from build123d import *

# Parameters (mm, degrees)
SKETCH1_W           = 80
SKETCH1_H           = 80
BOSS_EXTRUDE1_DEPTH = 5
SKETCH2_W           = 80
SKETCH2_H           = 5
BOSS_EXTRUDE2_DEPTH = 82
CUT_EXTRUDE1_DEPTH  = 81
CUT_EXTRUDE2_DEPTH  = 6
FILLET1_R           = 5
FILLET2_R           = 5
BOSS_EXTRUDE3_DEPTH = 80


with BuildPart() as part:
    # Sketch1 → Boss-Extrude1 (new body)
    with BuildSketch(Plane(origin=(0, 0, 0), x_dir=(1, 0, 0), z_dir=(0, 1, 0))):
        Rectangle(SKETCH1_W, SKETCH1_H)
    extrude(amount=BOSS_EXTRUDE1_DEPTH)

    # Sketch2 → Boss-Extrude2 (add)
    with BuildSketch(Plane(origin=(0, 5, 0), x_dir=(1, 0, 0), z_dir=(0, 1, 0))):
        with Locations((0, 37.5)):
            Rectangle(SKETCH2_W, SKETCH2_H)
    extrude(amount=BOSS_EXTRUDE2_DEPTH)

    # Sketch6 → Cut-Extrude1 (cut, through all)
    with BuildSketch(Plane(origin=(0, 0, -40), x_dir=(-1, 0, 0), z_dir=(0, 0, -1))):
        with BuildLine():
            Line((-30, 82), (30, 82))
            ThreePointArc((30, 82), (35, 77), (30, 72))
            Line((30, 72), (-30, 72))
            ThreePointArc((-30, 72), (-35, 77), (-30, 82))
        make_face()
        with BuildLine():
            Line((-30, 57), (30, 57))
            ThreePointArc((30, 57), (35, 52), (30, 47))
            Line((30, 47), (-30, 47))
            ThreePointArc((-30, 47), (-35, 52), (-30, 57))
        make_face()
    extrude(amount=-CUT_EXTRUDE1_DEPTH, mode=Mode.SUBTRACT)

    # Sketch7 → Cut-Extrude2 (cut, through all)
    with BuildSketch(Plane(origin=(0, 5, 0), x_dir=(1, 0, 0), z_dir=(0, 1, 0))):
        with BuildLine():
            Line((-35, -30), (-35, 15))
            ThreePointArc((-35, 15), (-30, 20), (-25, 15))
            Line((-25, 15), (-25, -30))
            ThreePointArc((-25, -30), (-30, -35), (-35, -30))
        make_face()
        with BuildLine():
            Line((35, 15), (35, -30))
            ThreePointArc((35, -30), (30, -35), (25, -30))
            Line((25, -30), (25, 15))
            ThreePointArc((25, 15), (30, 20), (35, 15))
        make_face()
    extrude(amount=-CUT_EXTRUDE2_DEPTH, mode=Mode.SUBTRACT)

    # Fillet1
    fillet1_edges = [part.edges().sort_by_distance(p)[0] for p in [
        (40, 2.5, 40),
        (-40, 2.5, 40),
    ]]
    fillet(fillet1_edges, radius=FILLET1_R)

    # Fillet2
    fillet2_edges = [part.edges().sort_by_distance(p)[0] for p in [
        (-40, 87, -37.5),
        (40, 87, -37.5),
    ]]
    fillet(fillet2_edges, radius=FILLET2_R)

    # Sketch8 → Boss-Extrude3 (add)
    with BuildSketch(Plane(origin=(40, 0, 0), x_dir=(0, 0, -1), z_dir=(1, 0, 0))):
        Polygon((35, 15), (25, 5), (35, 5), align=None)
    extrude(amount=-BOSS_EXTRUDE3_DEPTH)


solid = part.part
Check sheet for the modelled part. Datum: model origin and axes. Units: mm. A direction names the side the tool comes from. Round coordinates to 2 decimals unless told otherwise and drop trailing zeros. Write each loop counter-clockwise with the first axis right and the second up, starting at its lowest first coordinate (ties: lowest second). Pieces come first, ordered by that corner, then holes. Notation, with made-up numbers: (33, -12.75) -> (92, -12.75) arc R23 ccw to (92, 26.25) -> close; hole circle Ø1 at (76.25, 42). An arc over 180 degrees is marked (long way). Answer as CSV lines item,"result". Start each with the question number.
1) Section check D-D on x = 28.5. Enter the section's corners in (y, z).
2) Material ranges on line 1 (Z direction, x = -18, y = 61.5); line 2 (Y direction, x = 8, z = -0.5); line 3 (Y direction, x = -2, z = -28), recorded low to high. Write a range as from..to.
3) Tool access check on faces 5 (the flat face through (-35, 3, 8)), 6 (the flat face through (0, 82, -38)), 7 (the cylindrical face through (38, 86, -38)). Record the directions out of +Z, -Z, +X, -X, +Y, -Y that give a thin tool (end or side, any length) a straight path to the whole face; none if there is none.
4) Section check C-C on y = 52. Enter the section's corners in (x, z).
5) Section check B-B on z = 3.5. Enter the section's corners in (x, y).
6) Release check for a two-part mould opening along Z. For faces 1 (the cylindrical face through (30, 3, 35)), 2 (the flat face through (-1, 33, -40)), 3 (the flat face through (-25, 3, 7)), 4 (the flat face through (0, 47, -38)) record: pulls with the +Z half, pulls with the -Z half, needs draft (parallel to the pull), parting line crosses it, or undercut.
7) Section check A-A on x = -4.5. Enter the section's corners in (y, z), and give its area (3 significant figures).
8) Go/stop test with a flat-tipped pin: P1, Ø2, axis at x = 16, y = 30.5, coming from the +Z side. Record where the tip stops, or that it passes through.
Found:
1,outline,"(0, -40) -> (47, -40) -> (47, -35) -> (15, -35) -> (5, -25) -> (5, -19.77) -> (0, -19.77) -> close; (0, 34.77) -> (5, 34.77) -> (5, 40) -> (0, 40) -> close; (57, -40) -> (72, -40) -> (72, -35) -> (57, -35) -> close; (82, -40) -> (87, -40) -> (87, -35) -> (82, -35) -> close"
2,line 1,"z = -40..-35"
2,line 2,"y = 0..5"
2,line 3,"y = 0..8"
3,face 5,"+Y, -Y"
3,face 6,"+Z, -Z"
3,face 7,"+Z, -Z, +X, +Y"
4,outline,"(-40, -40) -> (-35, -40) -> (-35, -35) -> (-40, -35) -> close; (35, -40) -> (40, -40) -> (40, -35) -> (35, -35) -> close"
5,outline,"(-40, 0) -> (-35, 0) -> (-35, 5) -> (-40, 5) -> close; (-25, 0) -> (25, 0) -> (25, 5) -> (-25, 5) -> close; (35, 0) -> (40, 0) -> (40, 5) -> (35, 5) -> close"
6,face 1,"undercut"
6,face 2,"pulls with the -Z half"
6,face 3,"undercut"
6,face 4,"needs draft"
7,outline,"(0, -40) -> (47, -40) -> (47, -35) -> (15, -35) -> (5, -25) -> (5, 40) -> (0, 40) -> close; (57, -40) -> (72, -40) -> (72, -35) -> (57, -35) -> close; (82, -40) -> (87, -40) -> (87, -35) -> (82, -35) -> close"
7,area,"760 mm^2"
8,P1,"stops at z = -35"
